Model file for the job. Use its own axes, mm. Face numbers are marked on the shaded views. A direction names the side the tool comes from. Coordinates: 2 decimals unless noted, no trailing zeros. Order: outer loops, then holes, each group sorted by start corner. A loop starts at its lowest first (then second) coordinate and runs counter-clockwise, first axis right, second up. Notation, with made-up numbers: (56, 12) -> (106, 12) arc R15 cw to (106, 22) -> close; hole circle Ø5 at (6.5, 27.5). An arc over 180 degrees is marked (long way). Return JSON: item names as keys, results as strings. Group by question number.
1) Pull direction X, two halves, no side cores. Call the marked faces 1, 2 and 3: +X half, -X half, draft (parallel to the pull), parting line (faces both ways), or undercut.
2) Which spindle directions (+Z, -Z, +X, -X, +Y, -Y) get a long thin tool onto all of the face, cutting with end or side? Do the marked faces 4, 5 and 6. Say none if no direction does.
3) Flat gauge pins, fed straight in: pin 1 (13 mm diameter, centred on x = 16, y = 15.5, fed in from +Z); pin 2 (1.9 mm diameter, centred on x = -72.5, z = -68.5, fed in from +Y); pin 3 (2.5 mm diameter, centred on x = -24, y = 10.5, fed in from +Z). Where does each tip first touch, or does it go through?
4) Cut at B-B (x = -140). Write the cut outline in (y, z).
5) Cut at C-C (z = -61). Write the cut outline in (x, y).
6) Cut at D-D (x = -182). Write the cut outline in (y, z).
7) Probe line 1 (X direction, y = 16, z = -23.5); line 2 (Z direction, x = 23.5, y = 12.25); line 3 (X direction, y = 5, z = 0) (3 decimals). List the from-to ranges inside material, lowest first.
8) Cut at A-A (z = -23.5). Write the cut outline in (x, y).
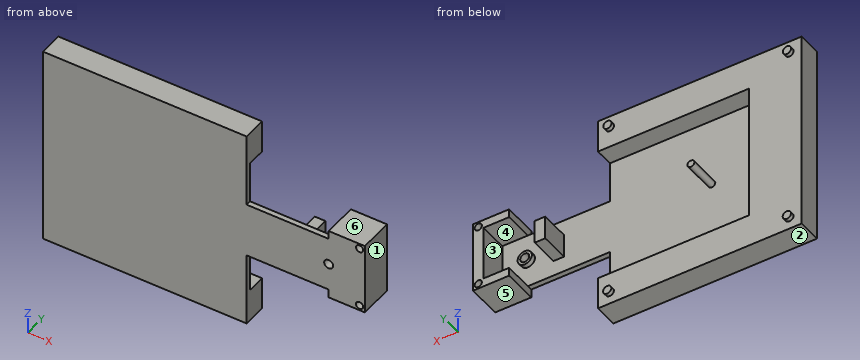
from build123d import *

# Parameters (mm, degrees)
SKETCH1_W           = 8
SKETCH1_H           = 18
SKETCH1_R           = 3.425
BOSS_EXTRUDE1_DEPTH = 4
SKETCH1_3_R         = 2.75
SKETCH1_3_W         = 8
SKETCH1_3_H         = 18
BOSS_EXTRUDE2_DEPTH = 25.9
SKETCH4_R           = 5.425
SKETCH4_R_2         = 3.425
BOSS_EXTRUDE5_DEPTH = 3.7
BOSS_EXTRUDE6_DEPTH = 14
SKETCH6_R           = 3.15
SKETCH6_R_2         = 3.175
BOSS_EXTRUDE7_DEPTH = 3
SKETCH7_R           = 2.65
BOSS_EXTRUDE8_DEPTH = 24.4


with BuildPart() as part:
    # Sketch1 → Boss-Extrude1 (new body)
    with BuildSketch(Plane(origin=(0, 0, 0), x_dir=(1, 0, 0), z_dir=(0, 1, 0))):
        Polygon((-62.5, -21), (0, -21), (19.5, -21), (19.5, 21), (0, 21), (-62.5, 21), (-62.5, 77.5), (-217.5, 77.5), (-217.5, -77.5), (-62.5, -77.5), align=None)
        with Locations((-23.5, 0)):
            Rectangle(SKETCH1_W, SKETCH1_H, mode=Mode.SUBTRACT)
        with Locations(Location((0, 0, 0), (0, 0, 270))):
            Circle(SKETCH1_R, mode=Mode.SUBTRACT)
    extrude(amount=BOSS_EXTRUDE1_DEPTH)

    # Sketch1_3 → Boss-Extrude2 (add)
    # profile 1 of 2: a face of its own
    with BuildSketch(Plane(origin=(0, 0, 0), x_dir=(1, 0, 0), z_dir=(0, 1, 0))):
        Polygon((27.5, -27.5), (27.5, 27.5), (0, 27.5), (0, 21), (19.5, 21), (19.5, -21), (0, -21), (0, -27.5), align=None)
        with Locations(Location((23.5, 23.5, 0), (0, 0, 90))):
            Circle(SKETCH1_3_R, mode=Mode.SUBTRACT)
        with Locations(Location((23.5, -23.5, 0), (0, 0, 90))):
            Circle(SKETCH1_3_R, mode=Mode.SUBTRACT)
    # profile 2 of 2: a face of its own
    with BuildSketch(Plane(origin=(0, 0, 0), x_dir=(1, 0, 0), z_dir=(0, 1, 0))):
        with Locations((-23.5, 0)):
            Rectangle(SKETCH1_3_W, SKETCH1_3_H)
    extrude(amount=BOSS_EXTRUDE2_DEPTH)

    # Sketch4 → Boss-Extrude5 (add)
    with BuildSketch(Plane(origin=(0, 4, 0), x_dir=(1, 0, 0), z_dir=(0, 1, 0))):
        with Locations(Location((0, 0, 0), (0, 0, 270))):
            Circle(SKETCH4_R)
        with Locations(Location((0, 0, 0), (0, 0, 270))):
            Circle(SKETCH4_R_2, mode=Mode.SUBTRACT)
    extrude(amount=BOSS_EXTRUDE5_DEPTH)

    # Sketch5 → Boss-Extrude6 (add)
    with BuildSketch(Plane(origin=(0, 4, 0), x_dir=(1, 0, 0), z_dir=(0, 1, 0))):
        Polygon((-217.5, 77.5), (-62.5, 77.5), (-62.5, 52.5), (-177.5, 52.5), (-177.5, -52.5), (-62.5, -52.5), (-62.5, -77.5), (-217.5, -77.5), align=None)
    extrude(amount=BOSS_EXTRUDE6_DEPTH)

    # Sketch6 → Boss-Extrude7 (add)
    with BuildSketch(Plane(origin=(0, 18, 0), x_dir=(1, 0, 0), z_dir=(0, 1, 0))):
        with Locations(Location((-71.48, 68.23, 0), (0, 0, 90))):
            Circle(SKETCH6_R)
        with Locations(Location((-71.61, -68.43, 0), (0, 0, 90))):
            Circle(SKETCH6_R)
        with Locations(Location((-208.29, -68.29, 0), (0, 0, 90))):
            Circle(SKETCH6_R)
        with Locations(Location((-208.265, 68.315, 0), (0, 0, 90))):
            Circle(SKETCH6_R_2)
    extrude(amount=BOSS_EXTRUDE7_DEPTH)

    # Sketch7 → Boss-Extrude8 (add)
    with BuildSketch(Plane(origin=(0, 4, 0), x_dir=(1, 0, 0), z_dir=(0, 1, 0))):
        with Locations(Location((-140, 0, 0), (0, 0, 270))):
            Circle(SKETCH7_R)
    extrude(amount=BOSS_EXTRUDE8_DEPTH)


solid = part.part
Answers below:
{
 "1": {"face 1": "+X half", "face 2": "draft", "face 3": "undercut"},
 "2": {"face 4": "+Y", "face 5": "-Z, +X, +Y, -Y", "face 6": "+Z, +X, +Y, -Y"},
 "3": {"pin 1": "stops at z = 27.5", "pin 2": "stops at y = 21", "pin 3": "stops at z = 9"},
 "4": {"outline": "(0, -77.5) -> (18, -77.5) -> (18, -52.5) -> (4, -52.5) -> (4, -2.65) -> (28.4, -2.65) -> (28.4, 2.65) -> (4, 2.65) -> (4, 52.5) -> (18, 52.5) -> (18, 77.5) -> (0, 77.5) -> close"},
 "5": {"outline": "(-217.5, 0) -> (-62.5, 0) -> (-62.5, 18) -> (-217.5, 18) -> close"},
 "6": {"outline": "(0, -77.5) -> (18, -77.5) -> (18, 77.5) -> (0, 77.5) -> close"},
 "7": {"line 1": "x = -217.5 to -177.5, 0 to 20.75, 26.25 to 27.5", "line 2": "z = -27.5 to -26.25, -20.75 to 20.75, 26.25 to 27.5", "line 3": "x = -217.5 to -177.5, -142.65 to -137.35, -27.5 to -19.5, -5.425 to -3.425, 3.425 to 5.425, 19.5 to 27.5"},
 "8": {"outline": "(-217.5, 0) -> (-62.5, 0) -> (-62.5, 4) -> (-177.5, 4) -> (-177.5, 18) -> (-217.5, 18) -> close; (0, 0) -> (20.75, 0) -> (20.75, 25.9) -> (0, 25.9) -> close; (26.25, 0) -> (27.5, 0) -> (27.5, 25.9) -> (26.25, 25.9) -> close"}
}
